Geometry: see drawing. Coordinates: mm, zero at the bounding-box minimum. A direction names the side the tool comes from. Coordinates: 2 decimals unless noted, no trailing zeros. Loops run counter-clockwise (first coordinate to the right, second up) from the corner with the lowest first, then second, coordinate; pieces in that order, holes last. Notation, with made-up numbers: (49, 20) - (75, 20) arc R26 cw to (75, 58) - close; hole circle Ø7 at (-24.75, 47). An arc over 180 degrees is marked (long way). Answer in a Markdown table with one row per item.
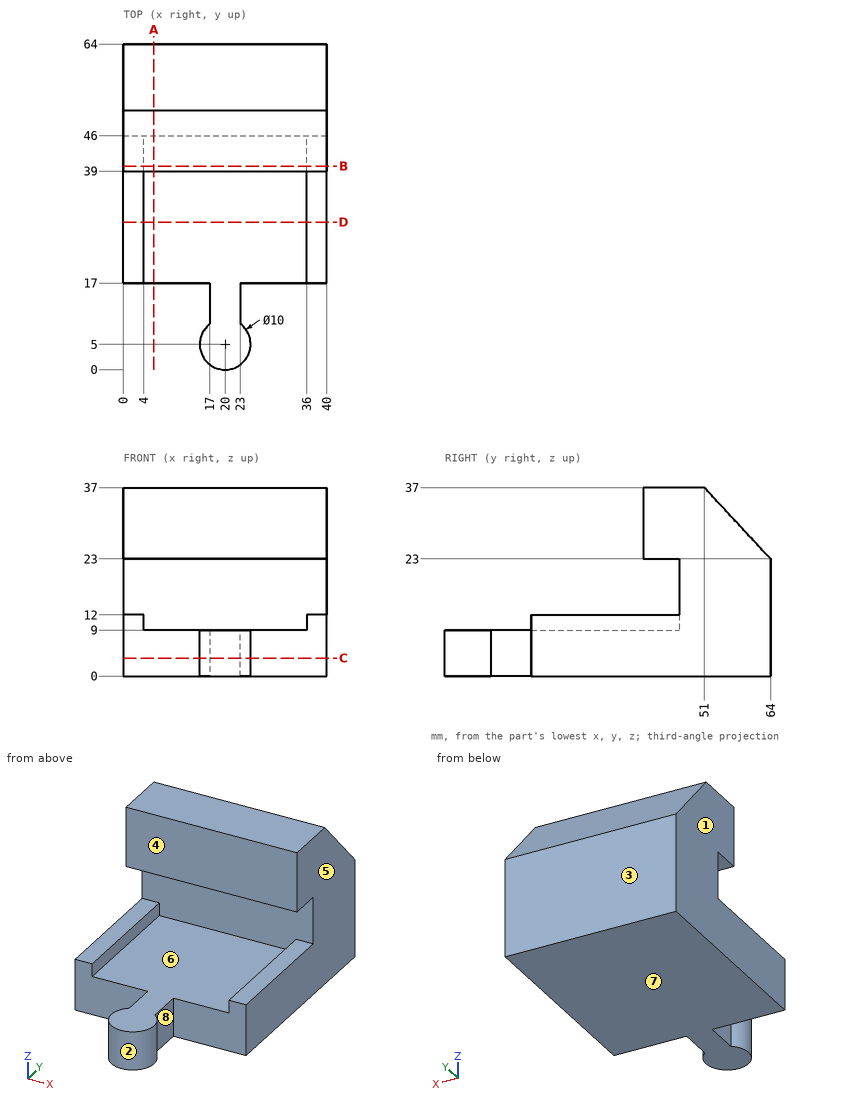
(1) First-contact query: pin 1 Ø7 at (x, z) = (20.5, 28) entering from -Y; pin 2 Ø8 at (x, y) = (8.5, 15) entering from +Z; pin 3 Ø8 at (y, z) = (44.5, 22) entering from -X; pin 4 Ø1.2 at (x, y) = (38.5, 27) entering from +Z. Flat tips, straight axial feed; report the tip coordinate or a pass-through.
Verdict:
| item | result |
|---|---|
| pin 1 | stops at y = 39 |
| pin 2 | stops at z = 9 |
| pin 3 | stops at x = 0 |
| pin 4 | stops at z = 12 |
(2) Ray query, probe 1 along X at (y, z) = (30, 11); probe 2 along Z at (x, y) = (21, 40); probe 3 along Y at (x, z) = (34, 11). Return the intervals inside material, ascending.
Verdict:
| item | result |
|---|---|
| probe 1 | x = 0 to 4, 36 to 40 |
| probe 2 | z = 0 to 9, 23 to 37 |
| probe 3 | y = 46 to 64 |
(3) Cut plane D-D on y = 29. Output: boundary loops of the cut face in (x, z).
Verdict:
| item | result |
|---|---|
| outline | (0, 0) - (40, 0) - (40, 12) - (36, 12) - (36, 9) - (4, 9) - (4, 12) - (0, 12) - close |
(4) Cut plane B-B on y = 40. Output: boundary loops of the cut face in (x, z).
Verdict:
| item | result |
|---|---|
| outline | (0, 0) - (40, 0) - (40, 12) - (36, 12) - (36, 9) - (4, 9) - (4, 12) - (0, 12) - close; (0, 23) - (40, 23) - (40, 37) - (0, 37) - close |
(5) Pull-direction query (Y, two-part tool) for the marked faces 1, 2 and 3; classes: pulls with the +Y half, pulls with the -Y half, needs draft (parallel to the pull), parting line crosses it, or undercut.
Verdict:
| item | result |
|---|---|
| face 1 | needs draft |
| face 2 | undercut |
| face 3 | pulls with the +Y half |
(6) Access query for the marked faces 4, 5, 6, 7 and 8. Directions: +Z, -Z, +X, -X, +Y, -Y. A direction counts if a zero-diameter tool reaches every point of the face in a straight line with its end or side. Return the directions, or none.
Verdict:
| item | result |
|---|---|
| face 4 | +Z, +X, -X, -Y |
| face 5 | +Z, -Z, +X, +Y, -Y |
| face 6 | -Y |
| face 7 | -Z, +X, -X, +Y, -Y |
| face 8 | +Z, -Z, +X |
(7) Cut plane A-A on x = 6. Output: boundary loops of the cut face in (y, z).
Verdict:
| item | result |
|---|---|
| outline | (17, 0) - (64, 0) - (64, 23) - (51, 37) - (39, 37) - (39, 23) - (46, 23) - (46, 9) - (17, 9) - close |
(8) Cut plane C-C on z = 3.5. Output: boundary loops of the cut face in (x, y), then the cut area to 3 significant figures.
Verdict:
| item | result |
|---|---|
| outline | (0, 17) - (17, 17) - (17, 9) arc R5 ccw (long way) to (23, 9) - (23, 17) - (40, 17) - (40, 64) - (0, 64) - close |
| area | 2,000 mm² |
